Design review of the part built by this model. Coordinates are the model's own, in mm. Face numbers are marked on the shaded views. Coordinates: 2 decimals unless noted, no trailing zeros. Order: outer loops, then holes, each group sorted by start corner. A loop starts at its lowest first (then second) coordinate and runs counter-clockwise, first axis right, second up. Notation, with made-up numbers: (38.25, -29.5) -> (63.25, -29.5) arc R20 ccw to (63.25, -9.5) -> close; hole circle Ø1 at (-29, 65). An arc over 180 degrees is marked (long way). Use a Markdown table: item, result. Add a question column.
Q1. Insertion check: pin 1 (1.1 mm diameter, centred on y = -22.5, z = 4, fed in from +X); pin 2 (2 mm diameter, centred on x = 3, y = -22.5, fed in from +Z); pin 3 (2 mm diameter, centred on x = -1.5, y = -8, fed in from +Z). Each pin has a flat end and moves straight along its axis. Give the tip position at first contact, or say it passes through.
Q2. Add section A-A (z = 0). State the section outline as (x, y) points (1 decimal).
Q3. The part is to be moulded in two halves that separate along X. For the marked faces 1, 2, 3 and 4, say which applies: pulls with the +X half, pulls with the -X half, needs draft (parallel to the pull), parting line crosses it, or undercut.
Q4. Add section C-C (y = -11.5). State the section outline as (x, z) points (1 decimal), then the cut area to 3 significant figures.
Q5. Wall thickness on probe 1 along Y at (x, z) = (3.5, -2.5) (1 decimal); probe 2 along Y at (x, z) = (-0.5, 4.5); probe 3 along X at (y, z) = (-18.5, -4): over which ranges is each line inside the solid? List them lowest first.
Q6. Add section D-D (z = 1.25). State the section outline as (x, y) points (1 decimal), then the cut area to 3 significant figures.
from build123d import *

# Parameters (mm, degrees)
F0_R            = 4.7625
F1_DEPTH        = 25.4
F2_W            = 3.175
F2_H            = 3.175
F3_DEPTH        = 6.35
F3_COPIES_COUNT = 2
F3_COPIES_PITCH = 19.05
F5_W            = 1.5875
F5_H            = 0.635


# Not quite as in the source:
# - a pattern or mirror of a feature is missing from the dataset's text; its kind, count and spacing are read off the source's solid


with BuildPart() as f1:
    # F0 (on Front) → F1 (new body)
    with BuildSketch(Plane.XZ):
        Circle(F0_R)
    extrude(amount=F1_DEPTH)

    # F2 (on face) → F3 (cut)
    with BuildSketch(Plane.XZ.offset(25.4)):
        with Locations((0, 4.7625)):
            Rectangle(F2_W, F2_H)
    f3 = extrude(amount=-F3_DEPTH, mode=Mode.SUBTRACT)

    # F3_copies: F3 ×2
    with Locations(*[(0, i * F3_COPIES_PITCH, 0) for i in range(1, F3_COPIES_COUNT)]):
        add(f3, mode=Mode.SUBTRACT)

    # F5 (on Right) → F6 (revolve, cut)
    with BuildSketch(Plane.YZ):
        with Locations((-23.01875, -4.445)):
            Rectangle(F5_W, F5_H)
    f6 = revolve(axis=Axis((0, -12.6913171262, 0), (0, 1, 0)), mode=Mode.SUBTRACT)

    # F6_copies: F6 across plane
    add(f6.mirror(Plane.ZX.offset(-12.7)), mode=Mode.SUBTRACT)


solid = f1.part
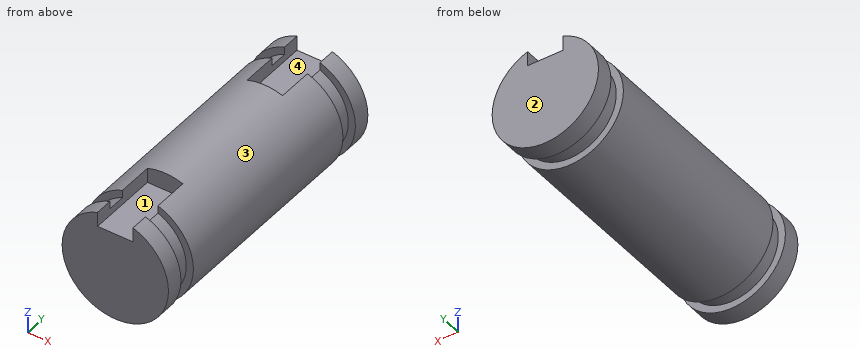
Established:
| question | item | result |
|---|---|---|
| 1 | pin 1 | x = 3.2 |
| 1 | pin 2 | z = 4.3 |
| 1 | pin 3 | z = 4.74 |
| 2 | outline | (-4.8, -25.4) -> (4.8, -25.4) -> (4.8, -23.8) -> (4.1, -23.8) -> (4.1, -22.2) -> (4.8, -22.2) -> (4.8, -3.2) -> (4.1, -3.2) -> (4.1, -1.6) -> (4.8, -1.6) -> (4.8, 0) -> (-4.8, 0) -> (-4.8, -1.6) -> (-4.1, -1.6) -> (-4.1, -3.2) -> (-4.8, -3.2) -> (-4.8, -22.2) -> (-4.1, -22.2) -> (-4.1, -23.8) -> (-4.8, -23.8) -> close |
| 3 | face 1 | undercut |
| 3 | face 2 | needs draft |
| 3 | face 3 | parting line crosses it |
| 3 | face 4 | undercut |
| 4 | outline | circle Ø9.5 at (0, 0) |
| 4 | area | 71.3 mm^2 |
| 5 | probe 1 | -25.4 to -23.8, -22.2 to -3.2, -1.6 to 0 |
| 5 | probe 2 | -19.05 to -6.35 |
| 5 | probe 3 | -2.58 to 2.58 |
| 6 | outline | (-4.6, -25.4) -> (4.6, -25.4) -> (4.6, -23.8) -> (3.9, -23.8) -> (3.9, -22.2) -> (4.6, -22.2) -> (4.6, -3.2) -> (3.9, -3.2) -> (3.9, -1.6) -> (4.6, -1.6) -> (4.6, 0) -> (-4.6, 0) -> (-4.6, -1.6) -> (-3.9, -1.6) -> (-3.9, -3.2) -> (-4.6, -3.2) -> (-4.6, -22.2) -> (-3.9, -22.2) -> (-3.9, -23.8) -> (-4.6, -23.8) -> close |
| 6 | area | 229 mm^2 |
